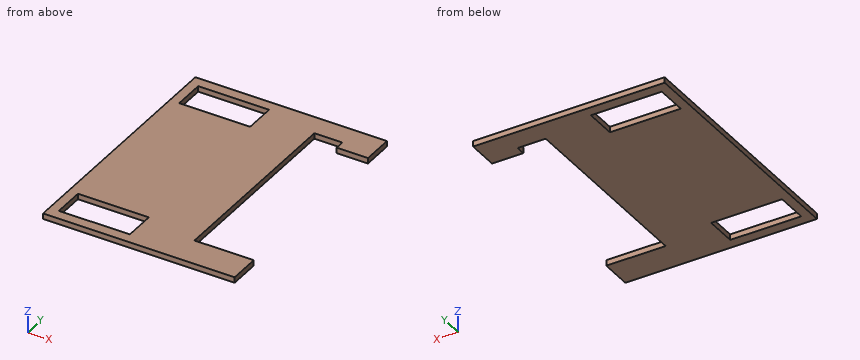
from build123d import *

# Parameters (mm, degrees)
SKETCH1_W           = 306.999208532
SKETCH1_H           = 400
SKETCH1_W_2         = 113.639208532
SKETCH1_H_2         = 50
BOSS_EXTRUDE1_DEPTH = 9
SKETCH2_W           = 95
SKETCH2_H           = 300
CUT_EXTRUDE1_DEPTH  = 460.151907085
SKETCH3_W           = 45
SKETCH3_H           = 15
CUT_EXTRUDE2_DEPTH  = 10


with BuildPart() as part:
    # Sketch1 → Boss-Extrude1 (new body)
    with BuildSketch(Plane.XY):
        with Locations((-170.312553906, 125.4)):
            Rectangle(SKETCH1_W, SKETCH1_H)
        with Locations((-251.992553906, 283.4)):
            Rectangle(SKETCH1_W_2, SKETCH1_H_2, mode=Mode.SUBTRACT)
        with Locations((-251.992553906, -32.6)):
            Rectangle(SKETCH1_W_2, SKETCH1_H_2, mode=Mode.SUBTRACT)
    extrude(amount=BOSS_EXTRUDE1_DEPTH)

    # Sketch2 → Cut-Extrude1 (cut, through all)
    with BuildSketch(Plane(origin=(0, 0, 0), x_dir=(-1, 0, 0), z_dir=(0, 0, -1))):
        with Locations((64.31294964, 125.4)):
            Rectangle(SKETCH2_W, SKETCH2_H)
    extrude(amount=-CUT_EXTRUDE1_DEPTH, mode=Mode.SUBTRACT)

    # Sketch3 → Cut-Extrude2 (cut)
    with BuildSketch(Plane(origin=(0, 0, 0), x_dir=(-1, 0, 0), z_dir=(0, 0, -1))):
        with Locations((89.31294964, 282.9)):
            Rectangle(SKETCH3_W, SKETCH3_H)
    extrude(amount=-CUT_EXTRUDE2_DEPTH, mode=Mode.SUBTRACT)


solid = part.part
CAD build for the part. Positions are in the model's coordinates, mm. Round coordinates to 2 decimals unless told otherwise and drop trailing zeros. Write each loop counter-clockwise with the first axis right and the second up, starting at its lowest first coordinate (ties: lowest second). Pieces come first, ordered by that corner, then holes.
(1) Slice it at A-A, the plane y = -12. Write the cut outline in (x, z), and give its area (3 significant figures).
(2) Slice it at B-B, the plane x = -248.5. Write the cut outline in (y, z).
(3) Slice it at D-D, the plane x = -98. Write the cut outline in (y, z), and give its area (3 significant figures).
(4) Drop a flat-ended pin along its axis: P1, Ø1, axis at y = 20, z = 6.5, coming from the +X side. Give the stop position or say it passes through.
(5) Slice it at C-C, the plane z = 1.75. Write the cut outline in (x, y), and give its area (3 significant figures).
(6) Probe line 1 along Y through (x, z) = (-217.5, 5.5); line 2 along Y through (x, z) = (-92.5, 0.5); line 3 along Y through (x, z) = (-64.5, 1.75). List the from-to ranges inside material, lowest first.
From the geometry:
1. outline: (-323.81, 0) - (-308.81, 0) - (-308.81, 9) - (-323.81, 9) - close; (-195.17, 0) - (-111.81, 0) - (-111.81, 9) - (-195.17, 9) - close
1. area: 885 mm2
2. outline: (-74.6, 0) - (-57.6, 0) - (-57.6, 9) - (-74.6, 9) - close; (-7.6, 0) - (258.4, 0) - (258.4, 9) - (-7.6, 9) - close; (308.4, 0) - (325.4, 0) - (325.4, 9) - (308.4, 9) - close
3. outline: (-74.6, 0) - (-24.6, 0) - (-24.6, 9) - (-74.6, 9) - close; (290.4, 0) - (325.4, 0) - (325.4, 9) - (290.4, 9) - close
3. area: 765 mm2
4. P1: stops at x = -111.81
5. outline: (-323.81, -74.6) - (-16.81, -74.6) - (-16.81, -24.6) - (-111.81, -24.6) - (-111.81, 290.4) - (-66.81, 290.4) - (-66.81, 275.4) - (-16.81, 275.4) - (-16.81, 325.4) - (-323.81, 325.4) - close; hole (-308.81, -57.6) - (-195.17, -57.6) - (-195.17, -7.6) - (-308.81, -7.6) - close; hole (-308.81, 258.4) - (-195.17, 258.4) - (-195.17, 308.4) - (-308.81, 308.4) - close
5. area: 82,300 mm2
6. line 1: y = -74.6 to -57.6, -7.6 to 258.4, 308.4 to 325.4
6. line 2: y = -74.6 to -24.6, 290.4 to 325.4
6. line 3: y = -74.6 to -24.6, 275.4 to 325.4
